Read the model definition and answer for the solid it produces. Units are mm, in the model's axes. A direction names the side the tool comes from. Coordinates: 2 decimals unless noted, no trailing zeros. Write each loop counter-clockwise with the first axis right and the second up, starting at its lowest first coordinate (ties: lowest second). Pieces come first, ordered by that corner, then holes. Notation, with made-up numbers: (32, 13.5) - (74, 13.5) arc R37 ccw to (74, 50.5) - close; hole circle Ø7 at (-4, 64.5). An arc over 180 degrees is marked (long way). Use a Markdown table: item, result.
from build123d import *

# Parameters (mm, degrees)
ESBO_O2_R                = 10
RESSALTO_EXTRUS_O1_DEPTH = 36
CORTE_EXTRUS_O1_REACH    = 38
ESBO_O3_R                = 1.6
CORTE_EXTRUS_O2_DEPTH    = 15


with BuildPart() as part:
    # Esboço2 → Ressalto-extrusão1 (new body)
    with BuildSketch(Plane.XY):
        Circle(ESBO_O2_R)
    extrude(amount=RESSALTO_EXTRUS_O1_DEPTH)

    # Esboço3 → Corte-extrusão1 (cut, up to next)
    with BuildSketch(Plane.XY.offset(36), mode=Mode.PRIVATE) as corte_extrus_o1_sk1:
        Circle(ESBO_O3_R)
    corte_extrus_o1_tool1 = extrude(corte_extrus_o1_sk1.sketch, amount=-CORTE_EXTRUS_O1_REACH, mode=Mode.PRIVATE) & part.part
    add(corte_extrus_o1_tool1.solids().sort_by_distance((0, 0, 36))[0], mode=Mode.SUBTRACT)

    # Esboço4 → Corte-extrusão2 (cut)
    with BuildSketch(Plane.XY.offset(36)):
        Polygon((0, 4.272391992), (-3.7, 2.136195996), (-3.7, -2.136195996), (0, -4.272391992), (3.7, -2.136195996), (3.7, 2.136195996), align=None)
    extrude(amount=-CORTE_EXTRUS_O2_DEPTH, mode=Mode.SUBTRACT)


solid = part.part
(1) Straight lines are drawn through the part: L1, parallel to Y at x = 0, z = 12.25; L2, parallel to Z at x = -1, y = -3; L3, parallel to X at y = 3.5, z = 26.5. For each, find the intervals that lie inside material, in ascending order.
Report:
| item | result |
|---|---|
| L1 | y = -10 to -1.6, 1.6 to 10 |
| L2 | z = 0 to 21 |
| L3 | x = -9.37 to -1.34, 1.34 to 9.37 |
(2) A cutting plane is placed at D-D, the plane z = 3. Write down the section's boundary in (x, y), and give its area (3 significant figures).
Report:
| item | result |
|---|---|
| outline | circle Ø20 at (0, 0); hole circle Ø3.2 at (0, 0) |
| area | 306 mm² |
(3) For faces 1 (the flat face through (1.876, 3.189, 28.605)), 2 (the flat face through (4, 0, 36)), determine the directions among +Z, -Z, +X, -X, +Y, -Y from which every point of the face is accessible in a straight line to the end or side of a thin tool.
Report:
| item | result |
|---|---|
| face 1 | +Z |
| face 2 | +Z, +X, -X, +Y, -Y |
(4) A cutting plane is placed at C-C, the plane x = -0.75. Write down the section's boundary in (y, z).
Report:
| item | result |
|---|---|
| outline | (-9.97, 0) - (-1.41, 0) - (-1.41, 21) - (-3.84, 21) - (-3.84, 36) - (-9.97, 36) - close; (1.41, 0) - (9.97, 0) - (9.97, 36) - (3.84, 36) - (3.84, 21) - (1.41, 21) - close |
(5) A cutting plane is placed at B-B, the plane z = 26.5. Write down the section's boundary in (x, y).
Report:
| item | result |
|---|---|
| outline | circle Ø20 at (0, 0); hole (-3.7, -2.14) - (0, -4.27) - (3.7, -2.14) - (3.7, 2.14) - (0, 4.27) - (-3.7, 2.14) - close |
(6) The mould has two halves that part along Y. Classify faces 3 (the flat face through (2, 0, 0)), 4 (the flat face through (3.7, 0, 29)), 5 (the cylindrical face through (-2.17, -9.76, 17.75)): pulls with the +Y half, pulls with the -Y half, needs draft (parallel to the pull), parting line crosses it, or undercut.
Report:
| item | result |
|---|---|
| face 3 | needs draft |
| face 4 | undercut |
| face 5 | parting line crosses it |
(7) A cutting plane is placed at A-A, the plane y = 0. Write down the section's boundary in (x, z).
Report:
| item | result |
|---|---|
| outline | (-10, 0) - (-1.6, 0) - (-1.6, 21) - (-3.7, 21) - (-3.7, 36) - (-10, 36) - close; (1.6, 0) - (10, 0) - (10, 36) - (3.7, 36) - (3.7, 21) - (1.6, 21) - close |
(8) Each of these flat-tipped pins is pushed along its axis until it touches: P1, Ø5, axis at y = 5, z = 14, coming from the +X side; P2, Ø10, axis at x = -5.5, z = 18.5, coming from the +Y side; P3, Ø1.5, axis at y = 4.5, z = 17, coming from the -X side. Where does it stop, or does it pass through?
Report:
| item | result |
|---|---|
| P1 | stops at x = 9.68 |
| P2 | stops at y = 9.99 |
| P3 | stops at x = -9.27 |
